from build123d import *

# Parameters (mm, degrees)
ESQUISSE1_R                    = 5.5
ESQUISSE1_R_2                  = 5
BOSS_EXTRU_1_DEPTH             = 28
BOSS_EXTRU_2_REACH             = 7.5
ESQUISSE2_R                    = 1
BOSS_EXTRU_2_DIRECTION_2_REACH = 7.5


with BuildPart() as part:
    # Esquisse1 → Boss.-Extru.1 (new body, symmetric)
    with BuildSketch(Plane.XY):
        Circle(ESQUISSE1_R)
        Circle(ESQUISSE1_R_2, mode=Mode.SUBTRACT)
    extrude(amount=BOSS_EXTRU_1_DEPTH, both=True)

    # Esquisse2 → Boss.-Extru.2 (add, up to next)
    with BuildSketch(Plane(origin=(0, 0, 0), x_dir=(1, 0, 0), z_dir=(0, 1, 0)), mode=Mode.PRIVATE) as boss_extru_2_sk1:
        with Locations((0, -19.5)):
            Circle(ESQUISSE2_R)
    boss_extru_2_tool1 = extrude(boss_extru_2_sk1.sketch, amount=BOSS_EXTRU_2_REACH, mode=Mode.PRIVATE) - part.part
    add(boss_extru_2_tool1.solids().sort_by_distance((0, 0, 19.5))[0])
    # Esquisse2 → Boss.-Extru.2 (add, up to next)
    with BuildSketch(Plane(origin=(0, 0, 0), x_dir=(1, 0, 0), z_dir=(0, 1, 0)), mode=Mode.PRIVATE) as boss_extru_2_sk2:
        with Locations((0, 27)):
            Circle(ESQUISSE2_R)
    boss_extru_2_tool2 = extrude(boss_extru_2_sk2.sketch, amount=BOSS_EXTRU_2_REACH, mode=Mode.PRIVATE) - part.part
    add(boss_extru_2_tool2.solids().sort_by_distance((0, 0, -27))[0])

    # Esquisse2 → Boss.-Extru.2 direction 2 (add, up to next)
    with BuildSketch(Plane(origin=(0, 0, 0), x_dir=(1, 0, 0), z_dir=(0, 1, 0)), mode=Mode.PRIVATE) as boss_extru_2_direction_2_sk1:
        with Locations((0, -19.5)):
            Circle(ESQUISSE2_R)
    boss_extru_2_direction_2_tool1 = extrude(boss_extru_2_direction_2_sk1.sketch, amount=-BOSS_EXTRU_2_DIRECTION_2_REACH, mode=Mode.PRIVATE) - part.part
    add(boss_extru_2_direction_2_tool1.solids().sort_by_distance((0, 0, 19.5))[0])
    # Esquisse2 → Boss.-Extru.2 direction 2 (add, up to next)
    with BuildSketch(Plane(origin=(0, 0, 0), x_dir=(1, 0, 0), z_dir=(0, 1, 0)), mode=Mode.PRIVATE) as boss_extru_2_direction_2_sk2:
        with Locations((0, 27)):
            Circle(ESQUISSE2_R)
    boss_extru_2_direction_2_tool2 = extrude(boss_extru_2_direction_2_sk2.sketch, amount=-BOSS_EXTRU_2_DIRECTION_2_REACH, mode=Mode.PRIVATE) - part.part
    add(boss_extru_2_direction_2_tool2.solids().sort_by_distance((0, 0, -27))[0])


solid = part.part
Geometry: final body of the model. Coordinates: model frame, mm. Give positions to 0.01 mm unless a question says otherwise; leave off trailing zeros. Write each loop counter-clockwise with the first axis right and the second up, starting at its lowest first coordinate (ties: lowest second). Pieces come first, ordered by that corner, then holes. Notation, with made-up numbers: M -2.5,73 L 6.5,73 A22 cw 6.5,111 Z; hole C 82.25,15 d4. An arc over 180 degrees is marked long. Answer in a Markdown table with one row per item. Add a question column.
(1) Mould query, pull axis Y, two halves, no side actions, for faces 1 (the cylindrical face through (-1.08, -4.88, -0.39)), 2 (the cylindrical face through (-1.19, -5.37, 0.39)), 3 (the flat face through (1.6, -4.9, -28)). Classes: +Y half, -Y half, draft (parallel to the pull), parting line (faces both ways), or undercut.
(2) Section A-A on y = 3.5. Return loops of the section in (x, z).
(3) Ray query, line 1 (Y direction, x = 0, z = -2.5); line 2 (X direction, y = 1.75, z = 12); line 3 (X direction, y = 4, z = -25). Return the intervals inside material, ascending.
(4) Section D-D on y = -2.75. Return loops of the section in (x, z).
(5) Section B-B on x = -3.75. Return loops of the section in (y, z), and give its area (3 significant figures).
(6) Section C-C on z = -27. Return loops of the section in (x, y), and give its area (3 significant figures).
(7) First-contact query: pin 1 (3 mm diameter, centred on y = -2, z = -14.5, fed in from +X); pin 2 (1.5 mm diameter, centred on x = 2.5, y = 2.5, fed in from +Z); pin 3 (5 mm diameter, centred on x = -3, z = -9, fed in from +Y); pin 4 (2 mm diameter, centred on x = -4, z = 12, fed in from -Y). Flat tips, straight axial feed; report the tip coordinate or a pass-through.
Result set:
| question | item | result |
|---|---|---|
| 1 | face 1 | undercut |
| 1 | face 2 | parting line |
| 1 | face 3 | draft |
| 2 | outline | M -4.24,-28 L -3.57,-28 L -3.57,28 L -4.24,28 Z; C 0,-27 d2; C 0,19.5 d2; M 3.57,-28 L 4.24,-28 L 4.24,28 L 3.57,28 Z |
| 3 | line 1 | y = -5.5 to -5, 5 to 5.5 |
| 3 | line 2 | x = -5.21 to -4.68, 4.68 to 5.21 |
| 3 | line 3 | x = -3.77 to -3, 3 to 3.77 |
| 4 | outline | M -4.76,-28 L -4.18,-28 L -4.18,28 L -4.76,28 Z; C 0,-27 d2; C 0,19.5 d2; M 4.18,-28 L 4.76,-28 L 4.76,28 L 4.18,28 Z |
| 5 | outline | M -4.02,-28 L -3.31,-28 L -3.31,28 L -4.02,28 Z; M 3.31,-28 L 4.02,-28 L 4.02,28 L 3.31,28 Z |
| 5 | area | 80.2 mm^2 |
| 6 | outline | C 0,0 d11; hole M -1,-4.9 L -1,4.9 A5 ccw Z; hole M 1,-4.9 A5 ccw 1,4.9 Z |
| 6 | area | 36.4 mm^2 |
| 7 | pin 1 | stops at x = 5.48 |
| 7 | pin 2 | passes through |
| 7 | pin 3 | stops at y = 5.48 |
| 7 | pin 4 | stops at y = -4.61 |
